Part model, mm, in its own coordinate system. A direction names the side the tool comes from. Give positions to 0.01 mm unless a question says otherwise; leave off trailing zeros. Write each loop counter-clockwise with the first axis right and the second up, starting at its lowest first coordinate (ties: lowest second). Pieces come first, ordered by that corner, then holes.
Autodesk Inventor part; units mm, degrees
ref_plane "YZ Plane" through (0, 0, 0) normal (1, 0, 0) x (0, 1, 0)
ref_plane "XZ Plane" through (0, 0, 0) normal (0, 1, 0) x (-1, 0, 0)
ref_plane "XY Plane" through (0, 0, 0) normal (0, 0, 1) x (1, 0, 0)
sketch "スケッチ1" plane through (0, 0, 0) normal (0, 0, 1) x (1, 0, 0)
  circle A0 centre (5, 5) radius 1.55
  circle A1 centre (5, -5) radius 1.55
  line L0 (0, 0) -> (100, 0) construction
  circle A2 centre (100, 0) radius 1.55
  line L1 (0, 10) -> (0, -10)
  line L2 (0, -10) -> (10, -10)
  line L3 (10, -10) -> (100.266, -5.9941)
  line L4 (10, 10) -> (100.266, 5.9941)
  arc A3 (100.266, -5.9941) -> (100.266, 5.9941) centre (100, 0) ccw
  line L5 (94.942, -3.2274) -> (11, -6.9527)
  line L6 (94.942, 3.2274) -> (11, 6.9527)
  arc A4 (94.942, 3.2274) -> (94.942, -3.2274) centre (100, 0) ccw
  line L7 (11, -6.9527) -> (11, 6.9527)
  line L8 (5, -5) -> (5, 5)
  line L9 (0, 10) -> (10, 10)
  line L10 (7.76, 6.5935) -> (7.76, 3.4065)
  line L11 (7.76, 3.4065) -> (5, 1.813)
  line L12 (5, 1.813) -> (2.24, 3.4065)
  line L13 (2.24, 3.4065) -> (2.24, 6.5935)
  line L14 (2.24, 6.5935) -> (5, 8.187)
  line L15 (5, 8.187) -> (7.76, 6.5935)
  arc A5 (4.0907, 2.338) -> (5.9093, 2.338) centre (5, 2.863) ccw
  arc A6 (6.8507, 2.8815) -> (7.76, 4.4565) centre (6.8507, 3.9315) ccw
  arc A7 (7.76, 5.5435) -> (6.8507, 7.1185) centre (6.8507, 6.0685) ccw
  arc A8 (5.9093, 7.662) -> (4.0907, 7.662) centre (5, 7.137) ccw
  arc A9 (3.1493, 7.1185) -> (2.24, 5.5435) centre (3.1493, 6.0685) ccw
  arc A10 (2.24, 4.4565) -> (3.1493, 2.8815) centre (3.1493, 3.9315) ccw
  line L16 (7.76, -6.5935) -> (7.76, -3.4065)
  line L17 (7.76, -3.4065) -> (5, -1.813)
  line L18 (5, -1.813) -> (2.24, -3.4065)
  line L19 (2.24, -3.4065) -> (2.24, -6.5935)
  line L20 (2.24, -6.5935) -> (5, -8.187)
  line L21 (5, -8.187) -> (7.76, -6.5935)
  arc A11 (5.9093, -2.338) -> (4.0907, -2.338) centre (5, -2.863) ccw
  arc A12 (7.76, -4.4565) -> (6.8507, -2.8815) centre (6.8507, -3.9315) ccw
  arc A13 (6.8507, -7.1185) -> (7.76, -5.5435) centre (6.8507, -6.0685) ccw
  arc A14 (4.0907, -7.662) -> (5.9093, -7.662) centre (5, -7.137) ccw
  arc A15 (2.24, -5.5435) -> (3.1493, -7.1185) centre (3.1493, -6.0685) ccw
  arc A16 (3.1493, -2.8815) -> (2.24, -4.4565) centre (3.1493, -3.9315) ccw
  circle A17 centre (100, 0) radius 1.55
  line L22 (103.51, 2.0265) -> (103.51, -2.0265)
  line L23 (103.51, -2.0265) -> (100, -4.053)
  line L24 (100, -4.053) -> (96.49, -2.0265)
  line L25 (96.49, -2.0265) -> (96.49, 2.0265)
  line L26 (96.49, 2.0265) -> (100, 4.053)
  line L27 (100, 4.053) -> (103.51, 2.0265)
  arc A18 (99.0907, -3.528) -> (100.9093, -3.528) centre (100, -3.003) ccw
  arc A19 (102.6007, -2.5515) -> (103.51, -0.9765) centre (102.6007, -1.5015) ccw
  arc A20 (103.51, 0.9765) -> (102.6007, 2.5515) centre (102.6007, 1.5015) ccw
  arc A21 (100.9093, 3.528) -> (99.0907, 3.528) centre (100, 3.003) ccw
  arc A22 (97.3993, 2.5515) -> (96.49, 0.9765) centre (97.3993, 1.5015) ccw
  arc A23 (96.49, -0.9765) -> (97.3993, -2.5515) centre (97.3993, -1.5015) ccw
  line L28 (100, 4.053) -> (100, -4.053) construction
  point P0 (5, 0)
  point P1 (7.76, 3.4065)
  point P2 (7.76, 6.5935)
  point P3 (5, 8.187)
  point P4 (2.24, 6.5935)
  point P5 (2.24, 3.4065)
  point P6 (3.1493, 7.1185)
  point P7 (4.0907, 7.662)
  point P8 (6.8507, 7.1185)
  point P9 (7.76, 5.5435)
  point P10 (7.76, 4.4565)
  point P11 (6.8507, 2.8815)
  point P12 (6.8507, -2.8815)
  point P13 (7.76, -5.5435)
  point P14 (6.8507, -7.1185)
  point P15 (3.1493, -7.1185)
  point P16 (2.24, -4.4565)
  point P17 (3.1493, -2.8815)
  point P18 (96.49, 2.0265)
  point P19 (96.49, -2.0265)
  point P20 (102.6007, -2.5515)
  point P21 (97.3993, -2.5515)
  point P22 (96.49, -0.9765)
  point P23 (96.49, 0.9765)
  point P24 (97.3993, 2.5515)
  point P25 (99.0907, 3.528)
  point P26 (100.9093, 3.528)
  point P27 (102.6007, 2.5515)
  point P28 (103.51, 0.9765)
  point P29 (103.51, -0.9765)
  dimension "d0" = 10
  dimension "d1" = 3.1
  dimension "d2" = 3.1
  dimension "d3" = 100
  dimension "d4" = 6
  dimension "d33" = 3
  dimension "d34" = 6
  dimension "d35" = 6
  dimension "d40" = 20
  dimension "d41" = 5
  dimension "d42" = 10
  dimension "d43" = 5.52
  dimension "d44" = 2.1
  dimension "d47" = 360
  dimension "d57" = 3.1
  dimension "d58" = 7.02
  dimension "d59" = 2.1
  dimension "d60" = 360
extrude "押し出し1" add sketch "スケッチ1" along normal blind 5 contours L9 L4 A3 L3 L2 L1
extrude "押し出し5" add sketch "スケッチ1" along normal blind 3.5 contours L12 L13 L14 L15 L10 L11 | L11 A5 | A11 L17 | L17 L16 L21 L20 L19 L18 | L18 A11 | A5 L12 | L11 A6 | A10 L12 | A12 L17 | L18 A16 | L10 A6 | A10 L13 | A12 L16 | L19 A16 | L10 A7 | A9 L13 | A13 L16 | L19 A15 | L15 A7 | A9 L14 | A13 L21 | L20 A15 | L15 A8 | A8 L14 | A14 L21 | L20 A14
extrude "押し出し6" add sketch "スケッチ1" along normal blind 2 contours A20 L22 | L22 L23 L24 L25 L26 L27 | L27 A20 | A19 L22 | L27 A21 | A19 L23 | L26 A21 | A18 L23 | L26 A22 | A18 L24 | L25 A22 | A23 L24 | L25 A23
extrude "押し出し7" add sketch "スケッチ1" along normal blind 1 contours L5 L7 L6 A4
fillet "フィレット2" radius 2 6 edges at (11, 6.9527, 3) (11, -6.9527, 3) (94.942, 3.2274, 3) (94.942, -3.2274, 3) (0, -10, 2.5) (0, 10, 2.5)
properties part number "胴体_サブフレーム_1_12" material "アセタール樹脂、黒"
1) Two-plate mould, pull along Y, no slides. Class faces 3 (the face through (54.501, -8.025, 2.465)), 4 (the face through (101.478, -0.466, 0.986)), 5 (the face through (0.6, 9.43, 2.54)): +Y half, -Y half, draft (parallel to the pull), parting line (faces both ways), or undercut.
Answers follow:
face 3: -Y half
face 4: undercut
face 5: +Y half
2) Saw through at B-B, the plane y = 0. Write the cut outline in (x, z), then the cut area to 3 significant figures.
Answers follow:
outline: (0, 0) - (98.45, 0) - (98.45, 2) - (96.49, 2) - (96.49, 5) - (94, 5) - (94, 1) - (11, 1) - (11, 5) - (0, 5) - close; (101.55, 0) - (106, 0) - (106, 5) - (103.51, 5) - (103.51, 2) - (101.55, 2) - close
area: 171 mm2
3) Saw through at A-A, the plane x = 5. Write the cut outline in (y, z).
Answers follow:
outline: (-10, 0) - (-6.55, 0) - (-6.55, 3.5) - (-8.19, 3.5) - (-8.19, 5) - (-10, 5) - close; (-3.45, 0) - (3.45, 0) - (3.45, 3.5) - (1.81, 3.5) - (1.81, 5) - (-1.81, 5) - (-1.81, 3.5) - (-3.45, 3.5) - close; (6.55, 0) - (10, 0) - (10, 5) - (8.19, 5) - (8.19, 3.5) - (6.55, 3.5) - close
4) 3-axis set-ups, long thin cutter, end or side, ignore diameter. For faces 1 (the face through (3.7, -6.4, 3.5)), 2 (the face through (6, -10, 2)): which of +Z, -Z, +X, -X, +Y, -Y reach the whole face in a straight line?
Answers follow:
face 1: +Z
face 2: +Z, -Z, +X, -X, -Y
5) Pin check, flat tips, straight feed: pin 1 Ø1.9 at (x, y) = (100, 0) entering from -Z; pin 2 Ø1.7 at (x, y) = (4, 4) entering from +Z; pin 3 Ø1 at (x, z) = (25, 0.5) entering from +Y; pin 4 Ø1.5 at (x, z) = (12.5, 4) entering from -Y. Stop position of each tip, or through.
Answers follow:
pin 1: passes through
pin 2: stops at z = 3.5
pin 3: stops at y = 9.36
pin 4: stops at y = -9.92
6) Wall check: L1, parallel to Y at x = 5, z = 0.8; L2, parallel to Y at x = 100, z = 1.45; L3, parallel to X at y = -1.5, z = 2.65. Give the ranges that are in metal, low to high.
Answers follow:
L1: y = -10 to -6.55, -3.45 to 3.45, 6.55 to 10
L2: y = -6.01 to -1.55, 1.55 to 6.01
L3: x = 0 to 11, 94.11 to 96.35, 103.65 to 105.81
7) Saw through at D-D, the plane x = 47.5. Write the cut outline in (y, z).
Answers follow:
outline: (-8.34, 0) - (8.34, 0) - (8.34, 5) - (5.33, 5) - (5.33, 1) - (-5.33, 1) - (-5.33, 5) - (-8.34, 5) - close
8) Saw through at C-C, the plane z = 2.75. Count the separate pieces of the cut face and the enclosed holes in it, then the cut area to 3 significant figures.
Answers follow:
separate pieces: 1
enclosed holes: 4
area: 791 mm2
